Model file for the job. Use its own axes, mm. A direction names the side the tool comes from. Round coordinates to 2 decimals unless told otherwise and drop trailing zeros. Order: outer loops, then holes, each group sorted by start corner. A loop starts at its lowest first (then second) coordinate and runs counter-clockwise, first axis right, second up. Notation, with made-up numbers: (58.25, 25) -> (64.25, 25) arc R12 ccw to (64.25, 41) -> close; hole circle Ø11 at (27.25, 33). An arc over 180 degrees is marked (long way). Put each result on its own line as item: value. Start each with the question number.
Q1. Pull direction Y, two halves, no side cores. Call faces 4 (the face through (-4, -13, 0)), 5 (the face through (-10.433, 5.929, -55.303)), 6 (the face through (-2.539, -19.334, -2.774)), 7 (the face through (5.134, 9.87, -1.875)): released by +Y, released by -Y, zero draft, split by the parting line, or undercut.
Q2. Flat gauge pins, fed straight in: P1, Ø10, axis at x = -15.5, z = -15, coming from the +Y side; P2, Ø1.1, axis at x = 1.5, y = -13, coming from the -Z side; P3, Ø4, axis at y = -7, z = -21, coming from the -X side. Where does each tip first touch, or does it go through?
Q3. Probe L1, parallel to Y at x = 0, z = -32; L2, parallel to Y at x = 0, z = -14; L3, parallel to Z at x = -1, y = -5.5. List the from-to ranges inside material, lowest first.
Q4. Cut at C-C, the plane z = -32. List the corners of the cut face in (x, y).
Q5. Cut at A-A, the plane z = -49.5. List the corners of the cut face in (x, y).
Q6. 3-axis set-ups, long thin cutter, end or side, ignore diameter. For faces 1 (the face through (-8.787, 6.738, -28.143)), 2 (the face through (11, -6, -46)), 3 (the face through (0, 13, -46)): which of +Z, -Z, +X, -X, +Y, -Y reach the whole face in a straight line?
Q7. Cut at B-B, the plane z = -17.5. List the corners of the cut face in (x, y).
from build123d import *

# Parameters (mm, degrees)
SKETCH2_OUTSIDE_W  = 58.05
SKETCH2_OUTSIDE_H  = 58.05
CUT_EXTRUDE1_DEPTH = 19


with BuildPart() as part:
    # Sketch1 → Revolve1 (revolve)
    with BuildSketch(Plane(origin=(0, 0, 0), x_dir=(0, 0, -1), z_dir=(1, 0, 0)), mode=Mode.PRIVATE) as revolve1_sk:
        with BuildLine():
            Line((35, 0), (35, 11.7))
            ThreePointArc((35, 11.7), (34.765685425, 12.265685425), (34.2, 12.5))
            Line((34.2, 12.5), (30.943915758, 12.5))
            Line((30.943915758, 12.5), (28, 11))
            Line((28, 11), (2, 11))
            Line((2, 11), (0, 13))
            Line((0, 13), (0, 18.5))
            Line((0, 18.5), (1, 19.5))
            Line((1, 19.5), (4.5, 19.5))
            Line((4.5, 19.5), (5, 19))
            Line((5, 19), (5, 17.4))
            Line((5, 17.4), (8.65, 17.4))
            Line((8.65, 17.4), (8.65, 19))
            Line((8.65, 19), (9.15, 19.5))
            Line((9.15, 19.5), (39.85, 19.5))
            Line((39.85, 19.5), (46, 13.35))
            Line((46, 13.35), (63, 13.35))
            Line((63, 13.35), (65, 11.35))
            Line((65, 11.35), (65, 0))
            Line((65, 0), (35, 0))
        make_face()
    revolve(revolve1_sk.sketch.rotate(Axis((0, 0, 0), (0, 0, -1)), 90), axis=Axis((0, 0, 0), (0, 0, -1)))

    # Sketch2 outside → Cut-Extrude1 (cut)
    with BuildSketch(Plane(origin=(0, 0, -65), x_dir=(-1, 0, 0), z_dir=(0, 0, -1))):
        Rectangle(SKETCH2_OUTSIDE_W, SKETCH2_OUTSIDE_H)
        Polygon((-13.856406461, 0), (-6.92820323, -12), (6.92820323, -12), (13.856406461, 0), (6.92820323, 12), (-6.92820323, 12), align=None, mode=Mode.SUBTRACT)
    extrude(amount=-CUT_EXTRUDE1_DEPTH, mode=Mode.SUBTRACT)


solid = part.part
Ans:
1. face 4: zero draft
1. face 5: released by +Y
1. face 6: split by the parting line
1. face 7: undercut
2. P1: stops at y = 16.43
2. P2: stops at z = -46
2. P3: stops at x = -18.85
3. L1: y = -19.5 to -12.5, 12.5 to 19.5
3. L2: y = -19.5 to -11, 11 to 19.5
3. L3: z = -65 to -35
4. outline: circle Ø39 at (0, 0); hole circle Ø25 at (0, 0)
5. outline: (-13.32, -0.93) -> (-7.47, -11.07) arc R13.35 ccw to (-5.85, -12) -> (5.85, -12) arc R13.35 ccw to (7.47, -11.07) -> (13.32, -0.93) arc R13.35 ccw to (13.32, 0.93) -> (7.47, 11.07) arc R13.35 ccw to (5.85, 12) -> (-5.85, 12) arc R13.35 ccw to (-7.47, 11.07) -> (-13.32, 0.93) arc R13.35 ccw to start
6. face 1: none
6. face 2: -Z, +X, -Y
6. face 3: -Z, +X, -X, +Y
7. outline: circle Ø39 at (0, 0); hole circle Ø22 at (0, 0)
